The model under review builds one solid part; all positions refer to its coordinate system, in mm. A direction names the side the tool comes from. Coordinates: 2 decimals unless noted, no trailing zeros. Write each loop counter-clockwise with the first axis right and the second up, starting at its lowest first coordinate (ties: lowest second). Pieces come first, ordered by that corner, then holes. Notation, with made-up numbers: (54.25, 47) - (93.25, 47) arc R28 cw to (93.25, 81) - close; hole circle Ø3 at (-11.5, 6.5). An arc over 180 degrees is marked (long way). Use one line per item in the form item = value. Start each with the question number.
```python
from build123d import *

# Parameters (mm, degrees)
SKETCH1_R           = 12.7
BOSS_EXTRUDE1_DEPTH = 15.875
SKETCH2_R           = 15.875
BOSS_EXTRUDE2_DEPTH = 5.08
SKETCH3_W           = 60.96
SKETCH3_H           = 3.302
BOSS_EXTRUDE3_DEPTH = 5.08
SKETCH4_W           = 81.28
SKETCH4_H           = 23.622
BOSS_EXTRUDE4_DEPTH = 5.08
FILLET1_R           = 1.27
FILLET2_R           = 1.27
FILLET3_R           = 1.27
FILLET4_R           = 1.27
FILLET5_R           = 1.27
FILLET7_R           = 1.27
FILLET8_R           = 1.27
SKETCH6_R           = 7.8105
CUT_EXTRUDE1_DEPTH  = 3.175
SKETCH7_R           = 7.8105
CUT_EXTRUDE2_DEPTH  = 10.795
CUT_EXTRUDE2_TAPER  = 35.8


with BuildPart() as part:
    # Sketch1 → Boss-Extrude1 (new body)
    with BuildSketch(Plane(origin=(0, 0, 0), x_dir=(1, 0, 0), z_dir=(0, 1, 0))):
        with Locations(Location((0, 0, 0), (0, 0, 270))):
            Circle(SKETCH1_R)
    extrude(amount=BOSS_EXTRUDE1_DEPTH)

    # Sketch2 → Boss-Extrude2 (add)
    with BuildSketch(Plane(origin=(0, 15.875, 0), x_dir=(1, 0, 0), z_dir=(0, 1, 0))):
        with Locations(Location((0, 0, 0), (0, 0, 270))):
            Circle(SKETCH2_R)
    extrude(amount=BOSS_EXTRUDE2_DEPTH)

    # Sketch3 → Boss-Extrude3 (add)
    with BuildSketch(Plane(origin=(0, 20.955, 0), x_dir=(1, 0, 0), z_dir=(0, 1, 0))):
        Rectangle(SKETCH3_W, SKETCH3_H)
    extrude(amount=BOSS_EXTRUDE3_DEPTH)

    # Sketch4 → Boss-Extrude4 (add)
    with BuildSketch(Plane.XZ.offset(-20.955)):
        Rectangle(SKETCH4_W, SKETCH4_H)
    extrude(amount=BOSS_EXTRUDE4_DEPTH)

    # Fillet1
    fillet1_edges = [part.edges().sort_by_distance(p)[0] for p in [
        (30.48, 23.495, 1.651),
        (30.48, 23.495, -1.651),
        (-30.48, 23.495, -1.651),
        (-30.48, 23.495, 1.651),
    ]]
    fillet(fillet1_edges, radius=FILLET1_R)

    # Fillet2
    fillet2_edges = [part.edges().sort_by_distance(p)[0] for p in [
        (0, 26.035, 1.651),
        (-30.48, 26.035, 0),
        (30.48, 26.035, 0),
        (0, 26.035, -1.651),
        (30.108025612, 26.035, 1.279025612),
        (30.108025612, 26.035, -1.279025612),
        (-30.108025612, 26.035, -1.279025612),
        (-30.108025612, 26.035, 1.279025612),
    ]]
    fillet(fillet2_edges, radius=FILLET2_R)

    # Fillet3
    fillet3_edges = [part.edges().sort_by_distance(p)[0] for p in [
        (0, 20.955, -15.875),
        (0, 20.955, 15.875),
        (25.623675707, 20.955, 11.811),
        (-25.623675707, 20.955, 11.811),
        (-25.623675707, 20.955, -11.811),
        (25.623675707, 20.955, -11.811),
        (40.64, 20.955, 0),
        (-40.64, 20.955, 0),
    ]]
    fillet(fillet3_edges, radius=FILLET3_R)

    # Fillet4
    fillet4_edges = [part.edges().sort_by_distance(p)[0] for p in [
        (0, 15.875, -15.875),
        (0, 15.875, 15.875),
        (25.623675707, 15.875, -11.811),
        (40.64, 15.875, 0),
        (25.623675707, 15.875, 11.811),
        (-25.623675707, 15.875, 11.811),
        (-40.64, 15.875, 0),
        (-25.623675707, 15.875, -11.811),
    ]]
    fillet(fillet4_edges, radius=FILLET4_R)

    # Fillet5
    fillet5_edges = [part.edges().sort_by_distance(p)[0] for p in [
        (0, 15.875, -12.7),
    ]]
    fillet(fillet5_edges, radius=FILLET5_R)

    # Fillet7
    fillet7_edges = [part.edges().sort_by_distance(p)[0] for p in [
        (0, 0, -12.7),
    ]]
    fillet(fillet7_edges, radius=FILLET7_R)

    # Fillet8
    fillet8_edges = [part.edges().sort_by_distance(p)[0] for p in [
        (0, 20.955, 1.651),
        (-30.48, 20.955, 0),
        (0, 20.955, -1.651),
        (30.48, 20.955, 0),
        (-30.108025612, 20.955, 1.279025612),
        (-30.108025612, 20.955, -1.279025612),
        (30.108025612, 20.955, -1.279025612),
        (30.108025612, 20.955, 1.279025612),
    ]]
    fillet(fillet8_edges, radius=FILLET8_R)

    # Sketch6 → Cut-Extrude1 (cut)
    with BuildSketch(Plane.XZ):
        with Locations(Location((0, 0, 0), (0, 0, 270))):
            Circle(SKETCH6_R)
    extrude(amount=-CUT_EXTRUDE1_DEPTH, mode=Mode.SUBTRACT)

    # Sketch7 → Cut-Extrude2 (cut)
    with BuildSketch(Plane.XZ.offset(-3.175)):
        with Locations(Location((0, 0, 0), (0, 0, 270))):
            Circle(SKETCH7_R)
    extrude(amount=-CUT_EXTRUDE2_DEPTH, taper=CUT_EXTRUDE2_TAPER, mode=Mode.SUBTRACT)


solid = part.part
```
1. Take a section at B-B (y = 23.5). State the section outline as (x, z) points, plus the area to 3 significant figures.
2. For L1, parallel to X at y = 2.5, z = 0; L2, parallel to Y at x = -15.5, z = -9.5 (3 decimals); L3, parallel to Y at x = 4, z = 9.5 (3 decimals), list the stretches that pass through material, from the lowest coordinate up.
3. Take a section at A-A (x = 16). State the section outline as (y, z) points (3 decimals).
4. For faces 1 (the flat face through (25, 18, -11.811)), 2 (the flat face through (0, 23, -1.651)), 3 (the flat face through (25, 18, 11.811)), list the 3-axis set-ups (+Z, -Z, +X, -X, +Y, -Y) from which the entire face can be reached by the end or side of a thin tool; tool diameter is ignored.
5. Take a section at D-D (y = 5.75). State the section outline as (x, z) points, plus the area to 3 significant figures.
6. Take a section at C-C (y = 11.5). State the section outline as (x, z) points, plus the area to 3 significant figures.
7. For P1, Ø1.3, axis at x = -26.5, y = 19, coming from the -Z side; P2, Ø0.8, axis at x = 0.5, y = 23.5, coming from the +Z side; P3, Ø0.8, axis at x = -26.5, y = 18.5, coming from the +Z side, all flat-tipped, find the tip position at first contact; note any pin that passes through.
8. The part is to be moulded in two halves that separate along Z. For faces 4 (the cylindrical face through (-0.163, 18.397, 15.874)), 5 (the conical face through (-2.08, 11.05, 0.46)), 6 (the flat face through (-7.5, 0, -2.7)), 7 (the cylindrical face through (7.744, 1.565, 1.017)), say which applies: released by +Z, released by -Z, zero draft, split by the parting line, or undercut.
Returned:
q1.outline = (-30.48, -0.38) arc R1.27 ccw to (-29.21, -1.65) - (29.21, -1.65) arc R1.27 ccw to (30.48, -0.38) - (30.48, 0.38) arc R1.27 ccw to (29.21, 1.65) - (-29.21, 1.65) arc R1.27 ccw to (-30.48, 0.38) - close
q1.area = 200 mm²
q2.L1 = -12.7 to -7.81, 7.81 to 12.7
q2.L2 = 15.875 to 20.955
q2.L3 = 0 to 20.955
q3.outline = (15.875, -10.541) arc R1.27 ccw to (17.145, -11.811) - (19.685, -11.811) arc R1.27 ccw to (20.955, -10.541) - (20.955, -2.921) arc R1.27 cw to (22.225, -1.651) - (24.765, -1.651) arc R1.27 ccw to (26.035, -0.381) - (26.035, 0.381) arc R1.27 ccw to (24.765, 1.651) - (22.225, 1.651) arc R1.27 cw to (20.955, 2.921) - (20.955, 10.541) arc R1.27 ccw to (19.685, 11.811) - (17.145, 11.811) arc R1.27 ccw to (15.875, 10.541) - close
q4.face_1 = -Z, +X, +Y, -Y
q4.face_2 = -Z, +X, -X, +Y
q4.face_3 = +Z, +X, +Y, -Y
q5.outline = circle Ø25.4 at (0, 0); hole circle Ø11.91 at (0, 0)
q5.area = 395 mm²
q6.outline = circle Ø25.4 at (0, 0); hole circle Ø3.61 at (0, 0)
q6.area = 496 mm²
q7.P1 = -11.81
q7.P2 = 1.65
q7.P3 = 11.81
q8.face_4 = released by +Z
q8.face_5 = undercut
q8.face_6 = zero draft
q8.face_7 = undercut
